Build history of the part. All positions in model axes, mm. A direction names the side the tool comes from. Coordinates: 2 decimals unless noted, no trailing zeros. Write each loop counter-clockwise with the first axis right and the second up, starting at its lowest first coordinate (ties: lowest second). Pieces come first, ordered by that corner, then holes.
from build123d import *

# Parameters (mm, degrees)
F2_R      = 3
F2_W      = 1
F2_H      = 18
F3_DEPTH  = 4
F4_START  = 2
F2_R_2    = 1.75
F4_DEPTH  = 2
F2_W_2    = 10
F5_DEPTH  = 30
F6_START  = 26
F6_DEPTH  = 4
F7_R      = 8.125
F7_R_2    = 5
F8_DEPTH  = 10
F9_DEPTH  = 2
F10_START = 28
F10_DEPTH = 2
F11_SIZE  = 5
F12_SIZE  = 2
F13_R     = 1.5


# Not quite as in the source:
# - a feature names something its author has since deleted; it is built from what else it names


with BuildPart() as f3:
    # F2 (on Top) → F3 (new body)
    with BuildSketch(Plane.XY):
        Polygon((4, 11), (-4, 11), (-4, 9), (-4, -9), (-4, -11), (4, -11), align=None)
        with Locations((0, -7)):
            Circle(F2_R, mode=Mode.SUBTRACT)
        with Locations((0, 7)):
            Circle(F2_R, mode=Mode.SUBTRACT)
        with Locations((-4.5, 0)):
            Rectangle(F2_W, F2_H)
    extrude(amount=F3_DEPTH)

    # F2 (on Top) → F4 (join)
    with BuildSketch(Plane.XY.offset(F4_START)):
        with Locations((0, -7)):
            Circle(F2_R)
        with Locations((0, -7)):
            Circle(F2_R_2, mode=Mode.SUBTRACT)
        with Locations((0, 7)):
            Circle(F2_R)
        with Locations((0, 7)):
            Circle(F2_R_2, mode=Mode.SUBTRACT)
    extrude(amount=F4_DEPTH)

    # F2 (on Top) → F5 (join)
    with BuildSketch(Plane.XY):
        with Locations((-10, 0)):
            Rectangle(F2_W_2, F2_H)
    extrude(amount=F5_DEPTH)

    # F2 (on Top) → F6 (join)
    with BuildSketch(Plane.XY.offset(F6_START)):
        Polygon((4, 11), (-4, 11), (-4, 9), (-4, -9), (-4, -11), (4, -11), align=None)
        with Locations((0, -7)):
            Circle(F2_R, mode=Mode.SUBTRACT)
        with Locations((0, 7)):
            Circle(F2_R, mode=Mode.SUBTRACT)
        with Locations((-4.5, 0)):
            Rectangle(F2_W, F2_H)
    extrude(amount=F6_DEPTH)

    # F7 (on face) → F8 (cut)
    with BuildSketch(Plane(origin=(-15, 0, 0), x_dir=(0, -1, 0), z_dir=(-1, 0, 0))):
        with Locations((0, 15)):
            Circle(F7_R)
        with Locations((0, 15)):
            Circle(F7_R_2, mode=Mode.SUBTRACT)
        with Locations((0, 15)):
            Circle(F7_R_2)
    extrude(amount=-F8_DEPTH, mode=Mode.SUBTRACT)

    # F7 (on face) → F9 (join)
    with BuildSketch(Plane(origin=(-15, 0, 0), x_dir=(0, -1, 0), z_dir=(-1, 0, 0))):
        with Locations((0, 15)):
            Circle(F7_R)
        with Locations((0, 15)):
            Circle(F7_R_2, mode=Mode.SUBTRACT)
    extrude(amount=-F9_DEPTH)

    # F2 (on Top) → F10 (join)
    with BuildSketch(Plane.XY.offset(F10_START)):
        with Locations((0, 7)):
            Circle(F2_R)
        with Locations((0, 7)):
            Circle(F2_R_2, mode=Mode.SUBTRACT)
        with Locations((0, -7)):
            Circle(F2_R)
        with Locations((0, -7)):
            Circle(F2_R_2, mode=Mode.SUBTRACT)
    extrude(amount=F10_DEPTH)

    # F11
    f11_edges = [f3.edges().sort_by_distance(p)[0] for p in [
        (-15, 0, 0),
        (-15, 0, 30),
    ]]
    chamfer(f11_edges, length=F11_SIZE)

    # F12
    f12_edges = [f3.edges().sort_by_distance(p)[0] for p in [
        (-15, -9, 15),
        (-15, 9, 15),
        (-12.5, 9, 27.5),
        (-12.5, -9, 27.5),
        (-12.5, 9, 2.5),
        (-12.5, -9, 2.5),
    ]]
    chamfer(f12_edges, length=F12_SIZE)

    # F13
    f13_edges = [f3.edges().sort_by_distance(p)[0] for p in [
        (4, 11, 2),
        (4, -11, 2),
        (-4, -11, 2),
        (-4, 11, 2),
        (4, 11, 28),
        (-4, 11, 28),
        (-4, -11, 28),
        (4, -11, 28),
    ]]
    fillet(f13_edges, radius=F13_R)


solid = f3.part
(1) Two-plate mould, pull along X, no slides. Class faces 4 (the cylindrical face through (-0.38, -8.71, 28.99)), 5 (the flat face through (4, 0, 28)), 6 (the flat face through (-11.05, 7.99, 27.55)): pulls with the +X half, pulls with the -X half, needs draft (parallel to the pull), parting line crosses it, or undercut.
(2) Slice it at B-B, the plane y = 7.75. Give the number of separate pieces and of enclosed holes in the cut face, and give its area (3 significant figures).
(3) Slice it at D-D, the plane y = -2.75. List the corners of the cut face in (x, z), and give its area (3 significant figures).
(4) 3-axis set-ups, long thin cutter, end or side, ignore diameter. For faces 1 (the flat face through (-3, 0, 30)), 2 (the flat face through (0, -9, 28)), 3 (the flat face through (-13, 0.1, 9.7)): which of +Z, -Z, +X, -X, +Y, -Y reach the whole face in a straight line?
(5) Probe L1, parallel to Y at x = 0, z = 1.2; L2, parallel to Z at x = -3.5, y = -9.25; L3, parallel to Y at x = 0, z = 2.95. List the from-to ranges inside material, lowest first.
(6) Flat gauge pins, fed straight in: P1, Ø4, axis at x = -5.5, z = 17.5, coming from the +Y side; P2, Ø4.5, axis at x = -9, z = 13.5, coming from the -Y side; P3, Ø3, axis at x = 0, y = 7, coming from the +Z side; P4, Ø1.5, axis at y = -5, z = 17.5, coming from the +X side. Where does each tip first touch, or does it go through?
(7) Slice it at C-C, the plane x = -6. List the corners of the cut face in (y, z) (3 decimals).
(8) Slice it at A-A, the plane z = 15. List the corners of the cut face in (x, y) (3 decimals).
Results:
1. face 4: undercut
1. face 5: pulls with the +X half
1. face 6: pulls with the -X half
2. separate pieces: 3
2. enclosed holes: 0
2. area: 246 mm2
3. outline: (-15, 5) - (-10, 0) - (4, 0) - (4, 4) - (-5, 4) - (-5, 7.35) - (-13, 7.35) - (-13, 10.82) - (-15, 10.82) - close; (-15, 19.18) - (-13, 19.18) - (-13, 22.65) - (-5, 22.65) - (-5, 26) - (4, 26) - (4, 30) - (-10, 30) - (-15, 25) - close
3. area: 208 mm2
4. face 1: +Z, +X, -X, +Y, -Y
4. face 2: none
4. face 3: +X
5. L1: y = -11 to -10, -4 to 4, 10 to 11
5. L2: z = 0 to 4, 26 to 30
5. L3: y = -11 to -8.75, -5.25 to 5.25, 8.75 to 11
6. P1: stops at y = 9
6. P2: stops at y = -9
6. P3: passes through
6. P4: stops at x = -13
7. outline: (-9, 0) - (9, 0) - (9, 30) - (-9, 30) - close; hole circle Ø16.25 at (0, 15)
8. outline: (-15, -7) - (-13, -9) - (-5, -9) - (-5, -8.125) - (-13, -8.125) - (-13, -5) - (-15, -5) - close; (-15, 5) - (-13, 5) - (-13, 8.125) - (-5, 8.125) - (-5, 9) - (-13, 9) - (-15, 7) - close
